CAD build for the part. Positions are in the model's coordinates, mm. Face numbers are marked on the shaded views. Round coordinates to 2 decimals unless told otherwise and drop trailing zeros. Loops run counter-clockwise (first coordinate to the right, second up) from the corner with the lowest first, then second, coordinate; pieces in that order, holes last.
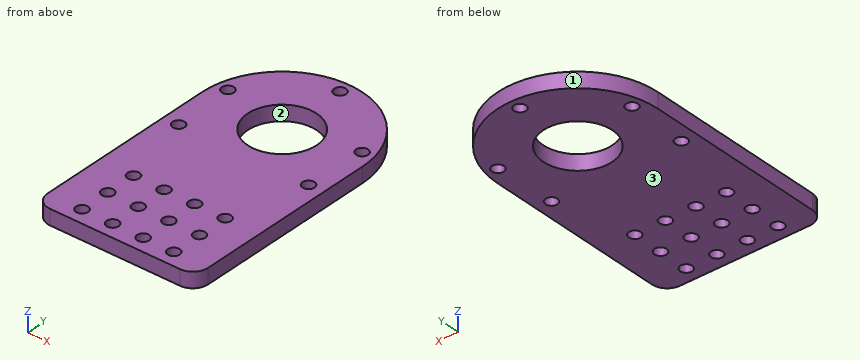
from build123d import *

# Parameters (mm, degrees)
SKETCH1_R           = 14.2875
SKETCH1_R_2         = 2.4892
BOSS_EXTRUDE1_DEPTH = 3.175
FILLET1_R           = 6.35


with BuildPart() as part:
    # Sketch1 → Boss-Extrude1 (new, symmetric)
    with BuildSketch(Plane.XY):
        with BuildLine():
            Line((33.3375, 0), (33.3375, -82.55))
            Line((33.3375, -82.55), (-33.3375, -82.55))
            Line((-33.3375, -82.55), (-33.3375, 0))
            ThreePointArc((-33.3375, 0), (0, 33.3375), (33.3375, 0))
        make_face()
        Circle(SKETCH1_R, mode=Mode.SUBTRACT)
        with Locations((-19.05, -76.2)):
            Circle(SKETCH1_R_2, mode=Mode.SUBTRACT)
        with Locations((-6.35, -76.2)):
            Circle(SKETCH1_R_2, mode=Mode.SUBTRACT)
        with Locations((-6.35, -63.5)):
            Circle(SKETCH1_R_2, mode=Mode.SUBTRACT)
        with Locations((-19.05, -63.5)):
            Circle(SKETCH1_R_2, mode=Mode.SUBTRACT)
        with Locations((6.35, -76.2)):
            Circle(SKETCH1_R_2, mode=Mode.SUBTRACT)
        with Locations((6.35, -63.5)):
            Circle(SKETCH1_R_2, mode=Mode.SUBTRACT)
        with Locations((-19.05, -50.8)):
            Circle(SKETCH1_R_2, mode=Mode.SUBTRACT)
        with Locations((-6.35, -50.8)):
            Circle(SKETCH1_R_2, mode=Mode.SUBTRACT)
        with Locations((6.35, -50.8)):
            Circle(SKETCH1_R_2, mode=Mode.SUBTRACT)
        with Locations((26.9875, -19.05)):
            Circle(SKETCH1_R_2, mode=Mode.SUBTRACT)
        with Locations((19.05, -76.2)):
            Circle(SKETCH1_R_2, mode=Mode.SUBTRACT)
        with Locations((19.05, -63.5)):
            Circle(SKETCH1_R_2, mode=Mode.SUBTRACT)
        with Locations((19.05, -50.8)):
            Circle(SKETCH1_R_2, mode=Mode.SUBTRACT)
        with Locations((0, 28.575)):
            Circle(SKETCH1_R_2, mode=Mode.SUBTRACT)
        with Locations((-27.86051193, 6.35)):
            Circle(SKETCH1_R_2, mode=Mode.SUBTRACT)
        with Locations((27.86051193, 6.35)):
            Circle(SKETCH1_R_2, mode=Mode.SUBTRACT)
        with Locations(Location((-26.9875, -19.05, 0), (0, 0, 180))):
            Circle(SKETCH1_R_2, mode=Mode.SUBTRACT)
    extrude(amount=BOSS_EXTRUDE1_DEPTH, both=True)

    # Fillet1
    fillet1_edges = [part.edges().sort_by_distance(p)[0] for p in [
        (33.3375, -82.55, 0),
        (-33.3375, -82.55, 0),
    ]]
    fillet(fillet1_edges, radius=FILLET1_R)


solid = part.part
Item 1: Cut at C-C (y = -50.8). List the corners of the cut face in (x, z) (1 decimal), plus the area to 3 significant figures.
Verdict:
outline: (-33.3, -3.2) - (-21.5, -3.2) - (-21.5, 3.2) - (-33.3, 3.2) - close; (-16.6, -3.2) - (-8.8, -3.2) - (-8.8, 3.2) - (-16.6, 3.2) - close; (-3.9, -3.2) - (3.9, -3.2) - (3.9, 3.2) - (-3.9, 3.2) - close; (8.8, -3.2) - (16.6, -3.2) - (16.6, 3.2) - (8.8, 3.2) - close; (21.5, -3.2) - (33.3, -3.2) - (33.3, 3.2) - (21.5, 3.2) - close
area: 297 mm2
Item 2: Flat gauge pins, fed straight in: P1, Ø5.5, axis at x = 19.05, y = -76.2, coming from the -Z side (3 decimals); P2, Ø3, axis at x = 6.35, y = -76.2, coming from the +Z side; P3, Ø3, axis at x = 8.5, z = -0.5, coming from the +Y side; P4, Ø1.5, axis at y = 9.5, z = -1.5, coming from the +X side. Where does each tip first touch, or does it go through?
Verdict:
P1: stops at z = -3.175
P2: passes through
P3: stops at y = 32.59
P4: stops at x = 32.17
Item 3: Cut at B-B (x = 0). State how many separate pieces and enclosed holes the cut face has, plus the area to 3 significant figures.
Verdict:
separate pieces: 3
enclosed holes: 0
area: 523 mm2
Item 4: Mould opens along Y. For the marked faces 1, 2 and 3 say: released by +Y, released by -Y, zero draft, split by the parting line, or undercut.
Verdict:
face 1: released by +Y
face 2: undercut
face 3: zero draft
Item 5: Wall check: L1, parallel to X at y = -51, z = 1.5; L2, parallel to Y at x = -6.35, z = -1; L3, parallel to Y at x = 28, z = 1. Give the ranges that are in metal, low to high.
Verdict:
L1: x = -33.34 to -21.53, -16.57 to -8.83, -3.87 to 3.87, 8.83 to 16.57, 21.53 to 33.34
L2: y = -82.55 to -78.69, -73.71 to -65.99, -61.01 to -53.29, -48.31 to -12.8, 12.8 to 32.73
L3: y = -82.47 to -21.32, -16.78 to 3.86, 8.84 to 18.09
Item 6: Cut at A-A (y = -19.05). List the corners of the cut face in (x, z) (1 decimal), plus the area to 3 significant figures.
Verdict:
outline: (-33.3, -3.2) - (-29.5, -3.2) - (-29.5, 3.2) - (-33.3, 3.2) - close; (-24.5, -3.2) - (24.5, -3.2) - (24.5, 3.2) - (-24.5, 3.2) - close; (29.5, -3.2) - (33.3, -3.2) - (33.3, 3.2) - (29.5, 3.2) - close
area: 360 mm2
Item 7: Cut at D-D (x = 19.05). List the corners of the cut face in (y, z) (3 decimals).
Verdict:
outline: (-82.55, -3.175) - (-78.689, -3.175) - (-78.689, 3.175) - (-82.55, 3.175) - close; (-73.711, -3.175) - (-65.989, -3.175) - (-65.989, 3.175) - (-73.711, 3.175) - close; (-61.011, -3.175) - (-53.289, -3.175) - (-53.289, 3.175) - (-61.011, 3.175) - close; (-48.311, -3.175) - (27.358, -3.175) - (27.358, 3.175) - (-48.311, 3.175) - close
